```python
from build123d import *

# Parameters (mm, degrees)
F0_W     = 76.2
F0_H     = 76.2
F0_W_2   = 63.5
F0_H_2   = 63.5
F1_DEPTH = 609.6
F3_D     = 12.7


# Not quite as in the source:
# - a length typed as a fraction of an inch, garbled in the dataset ("3 / 203.2 mm" for 3/8 in), is restored


with BuildPart() as f1:
    # F0 (on Top) → F1 (new body)
    with BuildSketch(Plane.XY):
        Rectangle(F0_W, F0_H)
        Rectangle(F0_W_2, F0_H_2, mode=Mode.SUBTRACT)
    extrude(amount=F1_DEPTH)

    # F3 (through all)
    with Locations(Plane.YZ.offset(38.1)):
        with Locations((0, 482.6)):
            Hole(F3_D / 2)


solid = f1.part
```
Geometry: final body of the model. Coordinates: model frame, mm. A direction names the side the tool comes from. Coordinates: 2 decimals unless noted, no trailing zeros. Loops run counter-clockwise (first coordinate to the right, second up) from the corner with the lowest first, then second, coordinate; pieces in that order, holes last. Notation, with made-up numbers: (72, -18.75) -> (91, -18.75) arc R27 cw to (91, 15.25) -> close; hole circle Ø1 at (89.5, 22.25). An arc over 180 degrees is marked (long way). Use a Markdown table: item, result. Add a question column.
(1) Section query A-A, the plane y = 26.5. Return loops of the section in (x, z).
(2) Mould query, pull axis Z, two halves, no side actions, for faces 3 (the flat face through (-34, 1, 0)), 4 (the cylindrical face through (-35, 0.8, 488.9)), 5 (the flat face through (-38.1, -1, 301)). Classes: pulls with the +Z half, pulls with the -Z half, needs draft (parallel to the pull), parting line crosses it, or undercut.
(3) Access query for faces 1 (the flat face through (-31.75, 0, 301)), 2 (the flat face through (-1, -38.1, 301)). Directions: +Z, -Z, +X, -X, +Y, -Y. A direction counts if a zero-diameter tool reaches every point of the face in a straight line with its end or side. Return the directions, or none.
(4) Section query C-C, the plane y = 0. Return loops of the section in (x, z), plus the area to 3 significant figures.
(5) Line query: line 1 along X through (y, z) = (-29, 128.5); line 2 along Z through (x, y) = (34, 0). Output: solid intervals per line, ascending.
(6) Section query D-D, the plane z = 468. Return loops of the section in (x, y), plus the area to 3 significant figures.
Answer:
| question | item | result |
|---|---|---|
| 1 | outline | (-38.1, 0) -> (-31.75, 0) -> (-31.75, 609.6) -> (-38.1, 609.6) -> close; (31.75, 0) -> (38.1, 0) -> (38.1, 609.6) -> (31.75, 609.6) -> close |
| 2 | face 3 | pulls with the -Z half |
| 2 | face 4 | undercut |
| 2 | face 5 | needs draft |
| 3 | face 1 | +Z, -Z |
| 3 | face 2 | +Z, -Z, +X, -X, -Y |
| 4 | outline | (-38.1, 0) -> (-31.75, 0) -> (-31.75, 476.25) -> (-38.1, 476.25) -> close; (-38.1, 488.95) -> (-31.75, 488.95) -> (-31.75, 609.6) -> (-38.1, 609.6) -> close; (31.75, 0) -> (38.1, 0) -> (38.1, 476.25) -> (31.75, 476.25) -> close; (31.75, 488.95) -> (38.1, 488.95) -> (38.1, 609.6) -> (31.75, 609.6) -> close |
| 4 | area | 7,580 mm^2 |
| 5 | line 1 | x = -38.1 to -31.75, 31.75 to 38.1 |
| 5 | line 2 | z = 0 to 476.25, 488.95 to 609.6 |
| 6 | outline | (-38.1, -38.1) -> (38.1, -38.1) -> (38.1, 38.1) -> (-38.1, 38.1) -> close; hole (-31.75, -31.75) -> (31.75, -31.75) -> (31.75, 31.75) -> (-31.75, 31.75) -> close |
| 6 | area | 1,770 mm^2 |
